Here's how the part is built. I have some questions about the finished solid (model axes, mm). Face numbers are marked on the shaded views. A direction names the side the tool comes from. Give positions to 0.01 mm unless a question says otherwise; leave off trailing zeros. Write each loop counter-clockwise with the first axis right and the second up, starting at its lowest first coordinate (ties: lowest second). Pieces come first, ordered by that corner, then holes. Notation, with made-up numbers: (-11, 88) - (27, 88) arc R30 ccw to (27, 116) - close; hole circle Ø1 at (47.25, -28.5). An arc over 180 degrees is marked (long way). Write each question's results on one line, items separated by ' | '. Start each with the question number.
Item 1: Please list where these lines run through material, in increasing order: line 1 along Y through (x, z) = (-2, 5); line 2 along X through (y, z) = (2.75, 0); line 3 along Z through (x, y) = (-2.5, 1.75).
Item 2: We'd pull the mould along Y, two halves only. Please class the marked faces 3, 4 and 5: +Y half, -Y half, draft (parallel to the pull), parting line (faces both ways), or undercut.
Item 3: Suppose I cut it at C-C on y = 3.25. List the corners of the cut face in (x, z) for me, then the cut area to 3 significant figures.
Item 4: Will these pins go through, and if not, where does the flat tip stop? P1, Ø3, axis at x = -2, y = 4, coming from the -Z side; P2, Ø1.5, axis at x = -2, y = 7, coming from the +Z side.
Item 5: Suppose I cut it at B-B on x = 0. List the corners of the cut face in (y, z) for me, then the cut area to 3 significant figures.
Item 6: Suppose I cut it at A-A on z = 0. List the corners of the cut face in (x, y) for me, then the cut area to 3 significant figures.
Item 7: Which directions (+Z, -Z, +X, -X, +Y, -Y) give clear straight access to the entire face, cutting with the end or side of a thin tool? Please do the marked faces 1 and 2.
Item 8: Suppose I cut it at D-D on x = -4. List the corners of the cut face in (y, z) for me, then the cut area to 3 significant figures.
```python
from build123d import *

# Parameters (mm, degrees)
ESQUISSE1_W        = 9.5
ESQUISSE1_H        = 11
BOSS_EXTRU_1_DEPTH = 7


with BuildPart() as part:
    # Esquisse1 → Boss.-Extru.1 (new body)
    with BuildSketch(Plane(origin=(0, 0, 0), x_dir=(1, 0, 0), z_dir=(0, 1, 0))):
        Rectangle(ESQUISSE1_W, ESQUISSE1_H)
    extrude(amount=-BOSS_EXTRU_1_DEPTH)

    # Esquisse3 → Révolution1 (revolve)
    with BuildSketch(Plane.XY, mode=Mode.PRIVATE) as r_volution1_sk:
        Polygon((0, 0), (0, 15), (3, 15), (3, 10), (2.5, 9.5), (2.5, 8), (3.5, 7), (3.5, 0), align=None)
    revolve(r_volution1_sk.sketch.rotate(Axis((0, 0, 0), (0, -1, 0)), 90), axis=Axis((0, 0, 0), (0, -1, 0)))


solid = part.part
```
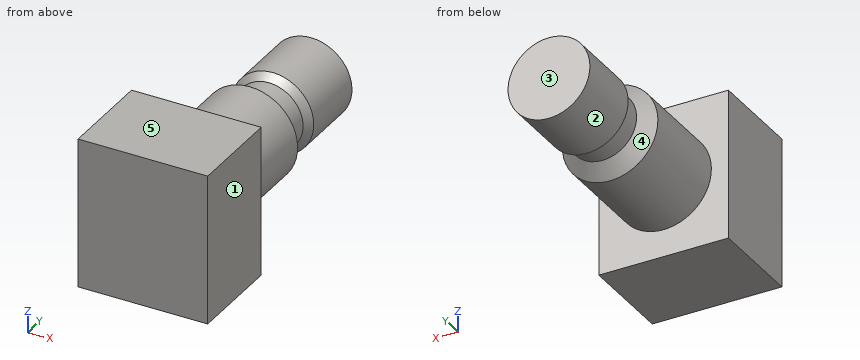
Checked values:
1) line 1: y = -7 to 0 | line 2: x = -3.5 to 3.5 | line 3: z = -2.45 to 2.45
2) face 3: +Y half | face 4: undercut | face 5: draft
3) outline: circle Ø7 at (0, 0) | area: 38.5 mm^2
4) P1: stops at z = -3.46 | P2: stops at z = 3.27
5) outline: (-7, -5.5) - (0, -5.5) - (0, -3.5) - (7, -3.5) - (8, -2.5) - (9.5, -2.5) - (10, -3) - (15, -3) - (15, 3) - (10, 3) - (9.5, 2.5) - (8, 2.5) - (7, 3.5) - (0, 3.5) - (0, 5.5) - (-7, 5.5) - close | area: 172 mm^2
6) outline: (-4.75, -7) - (4.75, -7) - (4.75, 0) - (3.5, 0) - (3.5, 7) - (2.5, 8) - (2.5, 9.5) - (3, 10) - (3, 15) - (-3, 15) - (-3, 10) - (-2.5, 9.5) - (-2.5, 8) - (-3.5, 7) - (-3.5, 0) - (-4.75, 0) - close | area: 162 mm^2
7) face 1: +Z, -Z, +X, +Y, -Y | face 2: +Y
8) outline: (-7, -5.5) - (0, -5.5) - (0, 5.5) - (-7, 5.5) - close | area: 77.0 mm^2
